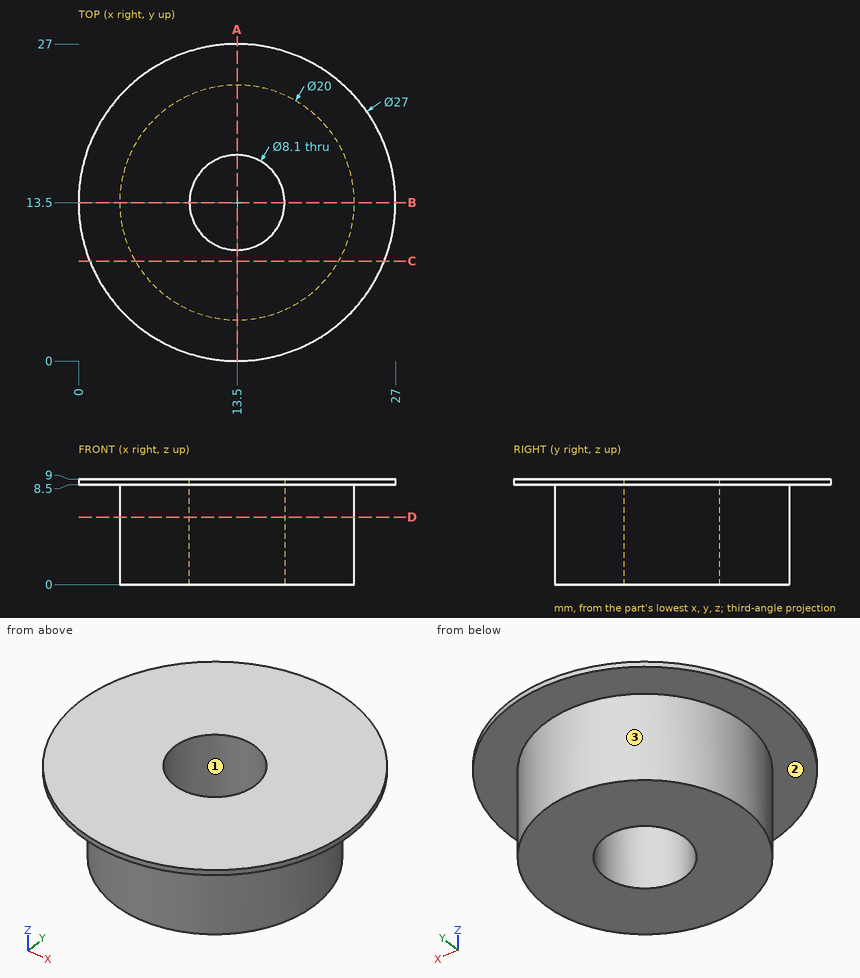
The figure shows three views and two pictorial views of one solid part (mm, origin at its lowest corner). Answer the questions. Round coordinates to 2 decimals unless told otherwise and drop trailing zeros. Order: outer loops, then holes, each group sorted by start corner. A loop starts at its lowest first (then second) coordinate and runs counter-clockwise, first axis right, second up.
Q1. Find the intervals of material crossed by line 1 along Y through (x, z) = (13.5, 7.25); line 2 along Z through (x, y) = (24.75, 9.5); line 3 along Y through (x, z) = (11, 8), in increasing order.
Solution:
line 1: y = 3.5 to 9.45, 17.55 to 23.5
line 2: z = 8.5 to 9
line 3: y = 3.82 to 10.31, 16.69 to 23.18
Q2. A cutting plane is placed at D-D, the plane z = 5.75. Determine the outline of the cut face in (x, y), then the cut area to 3 significant figures.
Solution:
outline: circle Ø20 at (13.5, 13.5); hole circle Ø8.1 at (13.5, 13.5)
area: 263 mm2
Q3. Given pin 1 Ø10.5 at (x, y) = (13.5, 13.5) entering from -Z; pin 2 Ø5 at (x, z) = (16.5, 5) entering from +Y; pin 3 Ø5 at (x, z) = (6, 2.5) entering from +Y; pin 4 Ø1 at (x, y) = (5.5, 24) entering from -Z, each flat-ended and moving along its own axis, determine where each tip first touches the part or whether it passes through.
Solution:
pin 1: stops at z = 0
pin 2: stops at y = 23.49
pin 3: stops at y = 22.16
pin 4: stops at z = 8.5
Q4. A cutting plane is placed at A-A, the plane x = 13.5. Determine the outline of the cut face in (y, z), then the cut area to 3 significant figures.
Solution:
outline: (0, 8.5) - (3.5, 8.5) - (3.5, 0) - (9.45, 0) - (9.45, 9) - (0, 9) - close; (17.55, 0) - (23.5, 0) - (23.5, 8.5) - (27, 8.5) - (27, 9) - (17.55, 9) - close
area: 111 mm2
Q5. The mould has two halves that part along X. Classify the marked faces 1, 2 and 3: pulls with the +X half, pulls with the -X half, needs draft (parallel to the pull), parting line crosses it, or undercut.
Solution:
face 1: undercut
face 2: needs draft
face 3: parting line crosses it
Q6. A cutting plane is placed at C-C, the plane y = 8.5. Determine the outline of the cut face in (x, z).
Solution:
outline: (0.96, 8.5) - (4.84, 8.5) - (4.84, 0) - (22.16, 0) - (22.16, 8.5) - (26.04, 8.5) - (26.04, 9) - (0.96, 9) - close
